```python
from build123d import *

# Parameters (mm, degrees)
F0_W     = 152.4
F0_H     = 50.8
F1_DEPTH = 76.2
F3_DEPTH = 92.964
F5_DEPTH = 93.472
F7_DEPTH = 203.454


with BuildPart() as f1:
    # F0 (on Front) → F1 (new body)
    with BuildSketch(Plane.XZ):
        with Locations((-76.2, 25.4)):
            Rectangle(F0_W, F0_H)
    extrude(amount=F1_DEPTH)

    # F2 (on face) → F3 (cut)
    with BuildSketch(Plane.XZ.offset(76.2)):
        Polygon((-101.6, 50.8), (-127, 50.8), (-127, 38.1), (-139.7, 38.1), (-139.7, 25.4), (-88.9, 25.4), (-88.9, 38.1), (-101.6, 38.1), align=None)
    extrude(amount=-F3_DEPTH, mode=Mode.SUBTRACT)

    # F4 (on face) → F5 (cut)
    with BuildSketch(Plane.XZ.offset(76.2)):
        Polygon((0, 50.8), (-76.2, 50.8), (-69.85, 38.1), (0, 38.1), align=None)
    extrude(amount=-F5_DEPTH, mode=Mode.SUBTRACT)

    # F6 (on face) → F7 (cut)
    with BuildSketch(Plane.YZ):
        Polygon((-63.5, 12.827001), (-50.8, 0), (-25.4, 0), (-12.7, 12.827001), align=None)
    extrude(amount=-F7_DEPTH, mode=Mode.SUBTRACT)


solid = f1.part
```
Verification items for the finished model (mm, model axes). A direction names the side the tool comes from. Coordinates: 2 decimals unless noted, no trailing zeros. Order: outer loops, then holes, each group sorted by start corner. A loop starts at its lowest first (then second) coordinate and runs counter-clockwise, first axis right, second up. Notation, with made-up numbers: (-9, 9.5) -> (48, 9.5) arc R31 ccw to (48, 37.5) -> close; hole circle Ø11 at (66.5, 18). An arc over 180 degrees is marked (long way). Answer as CSV lines item,"result". Start each with the question number.
1) Release check for a two-part mould opening along Z. For faces 1 (the face through (-152.4, -38, 25)), 2 (the face through (-115, -39, 25.4)), 3 (the face through (-89, -38, 50.8)) record: released by +Z, released by -Z, zero draft, split by the parting line, or undercut.
2) Cross-section at D-D, the plane y = -20.5. Record the boundary of the cut face in (x, z).
3) Material ranges on L1, parallel to X at y = -20.5, z = 32.5; L2, parallel to Z at x = -98.5, y = -7; L3, parallel to Z at x = -19.5, y = -43, recorded low to high. Write a range as [from, to].
4) Set-up check for faces 4 (the face through (-77, 0, 20)), 5 (the face through (-101.6, -39, 44)), 6 (the face through (-75, -38, 12.827)), 7 (the face through (-95, -39, 38.1)): record each of +Z, -Z, +X, -X, +Y, -Y from which the full face is reachable in a straight line by a thin tool's end or side.
5) Cross-section at B-B, the plane x = -128.5. Record the boundary of the cut face in (y, z), then the cut area to 3 significant figures.
6) Cross-section at C-C, the plane y = -70.5. Record the boundary of the cut face in (x, z), then the cut area to 3 significant figures.
7) Gauge pin test, flat ends, axial feed: pin 1 Ø10 at (y, z) = (-56, 23.5) entering from +X; pin 2 Ø6.5 at (x, y) = (-94.5, -41) entering from -Z; pin 3 Ø8 at (y, z) = (-58, 45.5) entering from +X; pin 4 Ø4 at (y, z) = (-40, 42) entering from +X. Record the tip position at first contact, or that the pin passes through.
8) Cross-section at A-A, the plane z = 42. Record the boundary of the cut face in (x, y), then the cut area to 3 significant figures.
Conclusion:
1,face 1,"zero draft"
1,face 2,"undercut"
1,face 3,"released by +Z"
2,outline,"(-152.4, 0) -> (0, 0) -> (0, 4.95) -> (-152.4, 4.95) -> close; (-152.4, 12.83) -> (0, 12.83) -> (0, 38.1) -> (-69.85, 38.1) -> (-76.2, 50.8) -> (-101.6, 50.8) -> (-101.6, 38.1) -> (-88.9, 38.1) -> (-88.9, 25.4) -> (-139.7, 25.4) -> (-139.7, 38.1) -> (-127, 38.1) -> (-127, 50.8) -> (-152.4, 50.8) -> close"
3,L1,"x = [-152.4, -139.7], [-88.9, 0]"
3,L2,"z = [0, 25.4], [38.1, 50.8]"
3,L3,"z = [12.83, 38.1]"
4,face 4,"+Z, -Z, +X, -X, +Y"
4,face 5,"+Z, +Y, -Y"
4,face 6,"+X, -X"
4,face 7,"+Y, -Y"
5,outline,"(-76.2, 0) -> (-50.8, 0) -> (-63.5, 12.83) -> (-12.7, 12.83) -> (-25.4, 0) -> (0, 0) -> (0, 25.4) -> (-76.2, 25.4) -> close; (-76.2, 38.1) -> (0, 38.1) -> (0, 50.8) -> (-76.2, 50.8) -> close"
5,area,"2,410 mm²"
6,outline,"(-152.4, 0) -> (0, 0) -> (0, 38.1) -> (-69.85, 38.1) -> (-76.2, 50.8) -> (-101.6, 50.8) -> (-101.6, 38.1) -> (-88.9, 38.1) -> (-88.9, 25.4) -> (-139.7, 25.4) -> (-139.7, 38.1) -> (-127, 38.1) -> (-127, 50.8) -> (-152.4, 50.8) -> close"
6,area,"5,850 mm²"
7,pin 1,"stops at x = 0"
7,pin 2,"stops at z = 12.83"
7,pin 3,"stops at x = -71.55"
7,pin 4,"stops at x = -70.8"
8,outline,"(-152.4, -76.2) -> (-127, -76.2) -> (-127, 0) -> (-152.4, 0) -> close; (-101.6, -76.2) -> (-71.8, -76.2) -> (-71.8, 0) -> (-101.6, 0) -> close"
8,area,"4,210 mm²"
